Can you work these out from the model? Positions are in its coordinate system, mm. A direction names the side the tool comes from. Give positions to 0.01 mm unless a question says otherwise; leave off trailing zeros. Write each loop counter-clockwise with the first axis right and the second up, starting at its lowest first coordinate (ties: lowest second). Pieces come first, ordered by that corner, then holes.
1. On a 3-axis mill with a long thin cutter (end or side, diameter ignored), from which of +Z, -Z, +X, -X, +Y, -Y can I reach the whole of each face in a straight line? I mean faces 5 (the cylindrical face through (14.3, -2, -0.1)), 6 (the flat face through (14.3, 0, -2.7)), 7 (the flat face through (5.2, 10, 0)). Say none if no direction works.
2. If I drill on probe 1 along Z at (x, y) = (9, 9.5); probe 2 along Y at (x, z) = (-14, -7), over which ranges is the centre line in solid material (lowest first)?
3. Thinking about a two-plate mould opening in Z: for faces 1 (the flat face through (0, 10, 5.2)), 2 (the flat face through (-5.2, 10, 0)), 3 (the cylindrical face through (-0.1, -2, -14.3)), 4 (the flat face through (6, -5, 0)), which applies, pulls with the +Z half, pulls with the -Z half, needs draft (parallel to the pull), parting line crosses it, or undercut?
4. Suppose I cut it at B-B (y = 17.5). Please give me the cut outline in (x, z).
5. Suppose I cut it at C-C (z = 0). Please give me the cut outline in (x, y).
6. Suppose I cut it at A-A (x = 0). Please give me the cut outline in (y, z), and give its area (3 significant figures).
7. I'm going to push flat-ended pins straight in: pin 1 (1.5 mm diameter, centred on x = 10.5, y = 15, fed in from -Z); pin 2 (6 mm diameter, centred on y = 6.5, z = -9.5, fed in from +X); pin 3 (4 mm diameter, centred on x = 7, y = 12.5, fed in from -Z); pin 4 (1 mm diameter, centred on x = 2.5, z = -3, fed in from +Y). Where does each tip first touch, or does it pass through?
```python
from build123d import *

# Parameters (mm, degrees)
SKETCH1_R           = 17.5
BOSS_EXTRUDE1_DEPTH = 25
SKETCH3_R           = 14.3
BOSS_EXTRUDE2_DEPTH = 5
SKETCH4_W           = 10.4
SKETCH4_H           = 10.4
CUT_EXTRUDE1_DEPTH  = 39.890872965
SKETCH6_R           = 2.1
CUT_EXTRUDE2_DEPTH  = 39.890872965
CHAMFER1_SIZE       = 0.363970234
CHAMFER1_SIZE_2     = 1


with BuildPart() as part:
    # Sketch1 → Boss-Extrude1 (new body)
    with BuildSketch(Plane(origin=(0, 0, 0), x_dir=(1, 0, 0), z_dir=(0, 1, 0))):
        with Locations(Location((0, 0, 0), (0, 0, 270))):
            Circle(SKETCH1_R)
    extrude(amount=BOSS_EXTRUDE1_DEPTH)

    # Sketch3 → Boss-Extrude2 (add)
    with BuildSketch(Plane.XZ):
        with Locations(Location((0, 0, 0), (0, 0, 90))):
            Circle(SKETCH3_R)
    extrude(amount=BOSS_EXTRUDE2_DEPTH)

    # Sketch4 → Cut-Extrude1 (cut, through all)
    with BuildSketch(Plane(origin=(0, 25, 0), x_dir=(1, 0, 0), z_dir=(0, 1, 0))):
        Rectangle(SKETCH4_W, SKETCH4_H)
    extrude(amount=-CUT_EXTRUDE1_DEPTH, mode=Mode.SUBTRACT)

    # Sketch6 → Cut-Extrude2 (cut, through all)
    with BuildSketch(Plane(origin=(0, 25, 0), x_dir=(1, 0, 0), z_dir=(0, 1, 0))):
        with Locations(Location((9, -9, 0), (0, 0, 270))):
            Circle(SKETCH6_R)
        with Locations(Location((-9, -9, 0), (0, 0, 270))):
            Circle(SKETCH6_R)
        with Locations(Location((-9, 9, 0), (0, 0, 270))):
            Circle(SKETCH6_R)
        with Locations(Location((9, 9, 0), (0, 0, 270))):
            Circle(SKETCH6_R)
    extrude(amount=-CUT_EXTRUDE2_DEPTH, mode=Mode.SUBTRACT)

    # Chamfer1
    # the kernel refuses this chamfer: 1, 0.363970234 mm, written as the material it takes off along each edge
    with BuildSketch(Plane(origin=(0, -5, 0), x_dir=(-0.7601968687413804, 0, 0.649692789521171), z_dir=(-0.649692789521171, 0, -0.7601968687413804))) as chamfer1_piece_1:
        Polygon((14.3 - CHAMFER1_SIZE, 0), (14.3, CHAMFER1_SIZE_2), (14.3, 0), align=None)
    revolve(axis=Axis((0, -5, 0), (0, 1, 0)), revolution_arc=98.963112953, mode=Mode.SUBTRACT)
    with BuildSketch(Plane(origin=(0, -5, 0), x_dir=(-0.6496927895211715, 0, 0.7601968687413799), z_dir=(0.7601968687413799, 0, 0.6496927895211715))) as chamfer1_piece_2:
        Polygon((14.3 - CHAMFER1_SIZE, 0), (14.3, -CHAMFER1_SIZE_2), (14.3, 0), align=None)
    revolve(axis=Axis((0, -5, 0), (0, -1, 0)), revolution_arc=98.963112953, mode=Mode.SUBTRACT)
    with BuildSketch(Plane(origin=(0, -5, 0), x_dir=(-0.7601968687413795, 0, -0.6496927895211719), z_dir=(-0.6496927895211719, 0, 0.7601968687413795))) as chamfer1_piece_3:
        Polygon((14.3, -CHAMFER1_SIZE_2), (14.3 - CHAMFER1_SIZE, 0), (14.3, 0), align=None)
    revolve(axis=Axis((0, -5, 0), (0, -1, 0)), revolution_arc=98.963112953, mode=Mode.SUBTRACT)
    with BuildSketch(Plane(origin=(0, -5, 0), x_dir=(0.6496927895211716, 0, -0.7601968687413798), z_dir=(-0.7601968687413798, 0, -0.6496927895211716))) as chamfer1_piece_4:
        Polygon((14.3, -CHAMFER1_SIZE_2), (14.3 - CHAMFER1_SIZE, 0), (14.3, 0), align=None)
    revolve(axis=Axis((0, -5, 0), (0, -1, 0)), revolution_arc=98.963112953, mode=Mode.SUBTRACT)


solid = part.part
```
Checks:
1. face 5: +X, -Y
1. face 6: -Y
1. face 7: +Y, -Y
2. probe 1: z = -15.01 to -11.1, -6.9 to 6.9, 11.1 to 15.01
2. probe 2: y = 0 to 25
3. face 1: undercut
3. face 2: undercut
3. face 3: pulls with the -Z half
3. face 4: needs draft
4. outline: circle Ø35 at (0, 0); hole circle Ø4.2 at (-9, -9); hole circle Ø4.2 at (-9, 9); hole (-5.2, -5.2) - (5.2, -5.2) - (5.2, 5.2) - (-5.2, 5.2) - close; hole circle Ø4.2 at (9, -9); hole circle Ø4.2 at (9, 9)
5. outline: (-17.5, 0) - (-14.3, 0) - (-14.3, -4) - (-13.94, -5) - (-5.2, -5) - (-5.2, 25) - (-17.5, 25) - close; (5.2, -5) - (13.94, -5) - (14.3, -4) - (14.3, 0) - (17.5, 0) - (17.5, 25) - (5.2, 25) - close
6. outline: (-5, -13.94) - (-4, -14.3) - (0, -14.3) - (0, -17.5) - (25, -17.5) - (25, -5.2) - (-5, -5.2) - close; (-5, 5.2) - (25, 5.2) - (25, 17.5) - (0, 17.5) - (0, 14.3) - (-4, 14.3) - (-5, 13.94) - close
6. area: 706 mm2
7. pin 1: stops at z = -14.53
7. pin 2: stops at x = 16.25
7. pin 3: stops at z = -16.77
7. pin 4: passes through
